Autodesk Inventor part; units mm, degrees
ref_plane "YZ Plane" through (0, 0, 0) normal (1, 0, 0) x (0, 1, 0)
ref_plane "XZ Plane" through (0, 0, 0) normal (0, 1, 0) x (-1, 0, 0)
ref_plane "XY Plane" through (0, 0, 0) normal (0, 0, 1) x (1, 0, 0)
sketch "Sketch1" plane through (0, 0, 0) normal (0, 1, 0) x (-1, 0, 0)
  line L0 (-15.5, -17.5) -> (15.5, -17.5)
  line L1 (17.5, -15.5) -> (17.5, 15.5)
  line L2 (15.5, 17.5) -> (-15.5, 17.5)
  line L3 (-17.5, 15.5) -> (-17.5, -15.5)
  line L4 (-17.5, -17.5) -> (17.5, 17.5) construction
  line L5 (17.5, -17.5) -> (-17.5, 17.5) construction
  line L6 (17.5, 15.5) -> (15.5, 17.5)
  line L7 (17.5, -15.5) -> (15.5, -17.5)
  line L8 (-15.5, -17.5) -> (-17.5, -15.5)
  line L9 (-15.5, 17.5) -> (-17.5, 15.5)
  point P0 (0, 0)
  dimension "d0" = 35
  dimension "d1" = 35
  dimension "d2" = 2
  dimension "d3" = 2
  dimension "d4" = 2
  dimension "d5" = 2
  dimension "d6" = 2
  dimension "d7" = 2
  dimension "d8" = 2
  dimension "d9" = 2
extrude "Extrusion1" add sketch "Sketch1" along normal blind 8
sketch "Sketch2" plane through (0, 8, 0) normal (0, 1, 0) x (1, 0, 0)
  line L0 (-17.5, -15.5) -> (-15.5, -17.5)
  line L1 (-15.5, -17.5) -> (15.5, -17.5)
  line L2 (15.5, -17.5) -> (17.5, -15.5)
  line L3 (17.5, -15.5) -> (17.5, 15.5)
  line L4 (17.5, 15.5) -> (15.5, 17.5)
  line L5 (15.5, 17.5) -> (-15.5, 17.5)
  line L6 (-15.5, 17.5) -> (-17.5, 15.5)
  line L7 (-17.5, 15.5) -> (-17.5, -15.5)
  line L8 (15.25, -17.25) -> (-15.25, -17.25)
  line L9 (-17.25, -15.25) -> (-17.25, 15.25)
  line L10 (-15.25, 17.25) -> (15.25, 17.25)
  line L11 (17.25, 15.25) -> (17.25, -15.25)
  line L12 (17.25, -17.25) -> (-17.25, 17.25) construction
  line L13 (-17.25, -17.25) -> (17.25, 17.25) construction
  line L14 (-17.25, 15.25) -> (-15.25, 17.25)
  line L15 (-17.25, -15.25) -> (-15.25, -17.25)
  line L16 (15.25, -17.25) -> (17.25, -15.25)
  line L17 (17.25, 15.25) -> (15.25, 17.25)
  point P0 (0, 0)
  dimension "d12" = 34.5
  dimension "d13" = 34.5
  dimension "d14" = 2
  dimension "d15" = 2
  dimension "d16" = 2
  dimension "d17" = 2
  dimension "d18" = 2
  dimension "d19" = 2
  dimension "d20" = 2
  dimension "d21" = 2
extrude "Extrusion2" add sketch "Sketch2" along normal blind 12 contours L8 L15 L9 L14 L10 L17 L11 L16
sketch "Sketch3" plane through (0, 20, 0) normal (0, 1, 0) x (1, 0, 0)
  line L0 (-17.5, -15.5) -> (-15.5, -17.5)
  line L1 (-17.5, 15.5) -> (-17.5, -15.5)
  line L2 (-15.5, 17.5) -> (-17.5, 15.5)
  line L3 (15.5, 17.5) -> (-15.5, 17.5)
  line L4 (17.5, 15.5) -> (15.5, 17.5)
  line L5 (17.5, -15.5) -> (17.5, 15.5)
  line L6 (15.5, -17.5) -> (17.5, -15.5)
  line L7 (-15.5, -17.5) -> (15.5, -17.5)
  point P0 (0, 0)
extrude "Extrusion3" add sketch "Sketch3" along normal blind 8
sketch "Sketch4" plane through (0, 28, 0) normal (0, 1, 0) x (1, 0, 0)
  circle A0 centre (0, 0) radius 11
  dimension "d26" = 22
extrude "Extrusion4" add sketch "Sketch4" along normal blind 2
sketch "Sketch5" plane through (0, 30, 0) normal (0, 1, 0) x (1, 0, 0)
  arc A0 (0.7737, 2.3773) -> (1.6586, -1.8706) centre (0, 0) ccw
  line L0 (1.6586, -1.8706) -> (0.7737, 2.3773)
  dimension "d29" = 5
extrude "Extrusion5" add sketch "Sketch5" along normal blind 22
sketch "Sketch6" plane through (0, 28, 0) normal (0, 1, 0) x (1, 0, 0)
  line L0 (15.5, 17.5) -> (-15.5, 17.5)
  line L1 (-17.5, 15.5) -> (-17.5, -15.5)
  line L2 (17.5, -15.5) -> (17.5, 15.5)
  line L3 (-15.5, -17.5) -> (15.5, -17.5)
  point P0 (0, 0)
  point P1 (-13, -13)
  point P2 (-13, 13)
  point P3 (13, 13)
  point P4 (13, -13)
  dimension "d32" = 26
  dimension "d33" = 26
  dimension "d34" = 4.5
  dimension "d35" = 4.5
  dimension "d45" = 4.5
  dimension "d46" = 4.5
  dimension "d47" = 4.5
  dimension "d48" = 4.5
  dimension "d49" = 4.5
hole "Hole1" at (-13, 28, 13) at (-13, 28, -13) at (13, 28, -13) at (13, 28, 13) direction (0, -1, 0) diameter 2.459 depth 8.8 tip angle 118
sketch "Sketch7" plane through (17.5, 0, 15.5) normal (1, 0, 0) x (0, 0, -1)
  line L0 (31, 0) -> (0, 0)
  line L1 (24.2568, 0) -> (6.5267, 0)
  line L2 (6.5267, 0) -> (6.5267, 3.8069)
  line L3 (6.5267, 3.8069) -> (24.2568, 3.8069)
  line L4 (24.2568, 3.8069) -> (24.2568, 0)
  point P0 (15.5, 0)
  point P1 (6.5267, 0)
extrude "Extrusion6" add sketch "Sketch7" along normal blind 3
equation "\"d3\" = d2"
equation "\"d4\" = d2"
equation "\"d5\" = d4"
equation "\"d6\" = d2"
equation "\"d7\" = d6"
equation "\"d8\" = d2"
equation "\"d9\" = d8"
equation "\"d15\" = d14"
equation "\"d16\" = d14"
equation "\"d17\" = d16"
equation "\"d18\" = d14"
equation "\"d19\" = d18"
equation "\"d20\" = d14"
equation "\"d21\" = d20"
properties part number "stepper"
Model file for the job. Use its own axes, mm. A direction names the side the tool comes from. Give positions to 0.01 mm unless a question says otherwise; leave off trailing zeros. Loops run counter-clockwise (first coordinate to the right, second up) from the corner with the lowest first, then second, coordinate; pieces in that order, holes last. Notation, with made-up numbers: (-34.75, -15.5) - (-2.75, -15.5) arc R31 ccw to (-2.75, 14.5) - close; hole circle Ø5 at (34, 58.25). An arc over 180 degrees is marked (long way). Use one line per item in the form item = value.
(1) Cut at B-B (y = 14.5). Give the cut face in (x, z), then the cut area to 3 significant figures.
Determined:
outline = (-17.25, -15.25) - (-15.25, -17.25) - (15.25, -17.25) - (17.25, -15.25) - (17.25, 15.25) - (15.25, 17.25) - (-15.25, 17.25) - (-17.25, 15.25) - close
area = 1,180 mm^2
(2) Cut at D-D (z = 7). Give the cut face in (x, y).
Determined:
outline = (-17.5, 0) - (20.5, 0) - (20.5, 3.81) - (17.5, 3.81) - (17.5, 8) - (17.25, 8) - (17.25, 20) - (17.5, 20) - (17.5, 28) - (8.49, 28) - (8.49, 30) - (-8.49, 30) - (-8.49, 28) - (-17.5, 28) - (-17.5, 20) - (-17.25, 20) - (-17.25, 8) - (-17.5, 8) - close
(3) Drill centre lines: L1, parallel to X at y = 24.75, z = -13; L2, parallel to Y at x = -8.5, z = 6.5. Where is each one in solid material? Low to high.
Determined:
L1 = -17.5 to -14.23, -11.77 to 11.77, 14.23 to 17.5
L2 = 0 to 30
(4) Drop flat-ended pins along their axis: P1, Ø2.5, axis at x = 19, y = 1.5, coming from the -Z side; P2, Ø3, axis at x = -2, y = 37, coming from the -Z side; P3, Ø3.5, axis at y = 14, z = 5, coming from the +X side. Give the stop position or say it passes through.
Determined:
P1 = -8.76
P2 = -2.45
P3 = 17.25
(5) Cut at C-C (x = 16.5). Give the cut face in (y, z).
Determined:
outline = (0, -16.5) - (8, -16.5) - (8, -16) - (20, -16) - (20, -16.5) - (28, -16.5) - (28, 16.5) - (20, 16.5) - (20, 16) - (8, 16) - (8, 16.5) - (0, 16.5) - close
(6) Cut at A-A (y = 23.5). Give the cut face in (x, z).
Determined:
outline = (-17.5, -15.5) - (-15.5, -17.5) - (15.5, -17.5) - (17.5, -15.5) - (17.5, 15.5) - (15.5, 17.5) - (-15.5, 17.5) - (-17.5, 15.5) - close; hole circle Ø2.46 at (-13, -13); hole circle Ø2.46 at (-13, 13); hole circle Ø2.46 at (13, -13); hole circle Ø2.46 at (13, 13)
(7) 3-axis set-ups, long thin cutter, end or side, ignore diameter. For faces 5 (the face through (12.631, 23.538, 14.173)), 6 (the face through (1.222, 40.846, -0.224)), 7 (the face through (17.5, 24, 0)), 8 (the face through (16.2, 13.9, 16.3)): which of +Z, -Z, +X, -X, +Y, -Y reach the whole face in a straight line?
Determined:
face_5 = +Y
face_6 = -Z, +X, +Y
face_7 = +Z, -Z, +X, +Y
face_8 = +Z, +X
(8) Pull direction Y, two halves, no side cores. Call faces 1 (the face through (2, 0, 0)), 2 (the face through (17.25, 14, 0)), 3 (the face through (-16, 24, -17)), 4 (the face through (19, 3.807, 0)): pulls with the +Y half, pulls with the -Y half, needs draft (parallel to the pull), parting line crosses it, or undercut.
Determined:
face_1 = pulls with the -Y half
face_2 = undercut
face_3 = needs draft
face_4 = pulls with the +Y half
